Can you work these out from the model? Positions are in its coordinate system, mm. Face numbers are marked on the shaded views. A direction names the side the tool comes from. Give positions to 0.01 mm unless a question says otherwise; leave off trailing zeros. Loops run counter-clockwise (first coordinate to the right, second up) from the corner with the lowest first, then second, coordinate; pieces in that order, holes last. Notation, with made-up numbers: (21, -36) - (56, -36) arc R28 ccw to (56, -17) - close; hole circle Ø4 at (38, -25.5). An arc over 180 degrees is marked (long way). Write item = value, one per line.
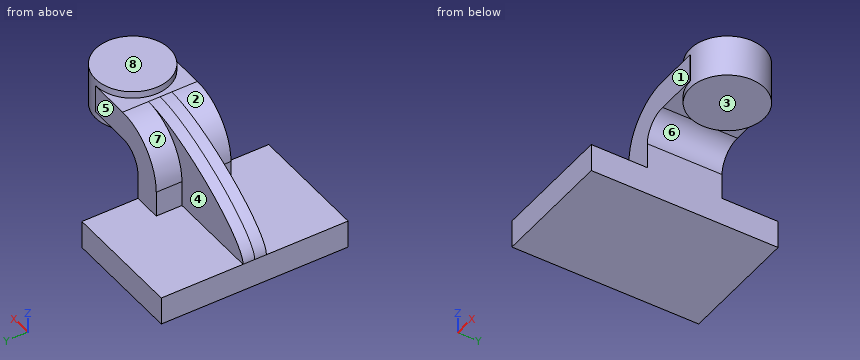
from build123d import *

# Parameters (mm, degrees)
F1_DEPTH = 63.5
F0_W     = 25.6068090757
F0_H     = 19.05
F2_DEPTH = 25.4
F3_DEPTH = 7.9375


with BuildPart() as f1:
    # F0 (on Front) → F1 (new body, symmetric)
    with BuildSketch(Plane.XZ):
        Polygon((-41.275, 9.525), (-41.275, -9.525), (41.275, -9.525), (41.275, 9.525), (22.225, 9.525), align=None)
    extrude(amount=F1_DEPTH, both=True)

    # F0 (on Front) → F2 (join, symmetric)
    with BuildSketch(Plane.XZ):
        with Locations((72.8420397361, 52.4002)):
            Rectangle(F0_W, F0_H)
        with BuildLine():
            Line((22.225, 9.525), (41.275, 9.525))
            Line((41.275, 9.525), (41.275, 27.0002))
            ThreePointArc((41.275, 27.0002), (45.9246798487, 38.2255201513), (57.15, 42.8752))
            Line((57.15, 42.8752), (60.0386351983, 42.8752))
            Line((60.0386351983, 42.8752), (60.0386351983, 61.9252))
            Line((60.0386351983, 61.9252), (57.15, 61.9252))
            ThreePointArc((57.15, 61.9252), (32.4542956671, 51.6959043329), (22.225, 27.0002))
            Line((22.225, 27.0002), (22.225, 9.525))
        make_face()
    extrude(amount=F2_DEPTH, both=True)

    # F0 (on Front) → F3 (join, symmetric)
    with BuildSketch(Plane.XZ):
        with BuildLine():
            add(Edge.make_bspline(
                [(-41.275, 9.525), (-41.275, 27.0002), (22.225, 61.9252), (57.15, 61.9252)],
                knots=[0, 0, 0, 0, 111.5045361635, 111.5045361635, 111.5045361635, 111.5045361635], degree=3))
            Line((-41.275, 9.525), (22.225, 9.525))
            Line((22.225, 9.525), (22.225, 27.0002))
            ThreePointArc((22.225, 27.0002), (32.4542956671, 51.6959043329), (57.15, 61.9252))
        make_face()
    extrude(amount=F3_DEPTH, both=True)

    # F0 (on Front) → F4 (revolve)
    with BuildSketch(Plane.XZ):
        Polygon((85.6454442739, 66.675), (85.6454442739, 61.9252), (85.6454442739, 42.8752), (85.6454442739, 38.1), (110.8386351983, 38.1), (110.8386351983, 66.675), align=None)
    revolve(axis=Axis((85.6454442739, 0, 52.3875), (0, 0, 1)))


solid = f1.part
Q1. Which directions (+Z, -Z, +X, -X, +Y, -Y) give clear straight access to the entire face, cutting with the end or side of a thin tool? Please do the marked faces 1, 2, 3, 4 and 5.
Output:
face_1 = +Z, +X, -X, -Y
face_2 = +Z, -X, -Y
face_3 = -Z, +X, +Y, -Y
face_4 = +Z, -X, +Y
face_5 = +Z, +X, -X, +Y
Q2. Imagine slicing it at C-C, the plane y = -45.5. Write out the boundary of the cut face in (x, z) (3 decimals), then the cut area to 3 significant figures.
Output:
outline = (-41.275, -9.525) - (41.275, -9.525) - (41.275, 9.525) - (-41.275, 9.525) - close
area = 1,570 mm2
Q3. For pin 1 (1 mm diameter, centred on x = -19.5, z = 16, fed in from +Y); pin 2 (8 mm diameter, centred on y = -4.5, z = 37.5, fed in from +X); pin 3 (12 mm diameter, centred on x = 78, y = 10, fed in from -Z), each with a flat end and sliding along its axis, tell me the tip position at first contact or that it passes through.
Output:
pin_1 = 7.94
pin_2 = 110.83
pin_3 = 38.1
Q4. I need wall thicknesses on L1, parallel to Z at x = -22, y = -22 (3 decimals); L2, parallel to Y at x = 30.5, z = 37.5; L3, parallel to Y at x = 1.5, z = 30.5. Which ranges of each line are inside material? Lowest first, please.
Output:
L1 = -9.525 to 9.525
L2 = -25.4 to 25.4
L3 = -7.94 to 7.94
Q5. We'd pull the mould along X, two halves only. Please class the marked faces 6, 7 and 8: released by +X, released by -X, zero draft, split by the parting line, or undercut.
Output:
face_6 = undercut
face_7 = released by -X
face_8 = zero draft
Q6. Imagine slicing it at B-B, the plane x = 75. Write out the boundary of the cut face in (y, z) (3 decimals).
Output:
outline = (-25.4, 42.875) - (-22.834, 42.875) - (-22.834, 38.1) - (22.834, 38.1) - (22.834, 42.875) - (25.4, 42.875) - (25.4, 61.925) - (22.834, 61.925) - (22.834, 66.675) - (-22.834, 66.675) - (-22.834, 61.925) - (-25.4, 61.925) - close
Q7. Imagine slicing it at A-A, the plane z = -1.5. Write out the boundary of the cut face in (x, y) (3 decimals), then the cut area to 3 significant figures.
Output:
outline = (-41.275, -63.5) - (41.275, -63.5) - (41.275, 63.5) - (-41.275, 63.5) - close
area = 10,500 mm2
